For this review, take the finished solid that the model builds, in its own axes (mm). A direction names the side the tool comes from. Round coordinates to 2 decimals unless told otherwise and drop trailing zeros. Order: outer loops, then holes, each group sorted by start corner. A loop starts at its lowest first (then second) coordinate and runs counter-clockwise, first axis right, second up. Notation, with made-up numbers: (-26.5, 49) -> (8.5, 49) arc R14 cw to (8.5, 71) -> close; hole circle Ø8 at (67.5, 22). An arc over 180 degrees is marked (long way). Use a Markdown table: item, result. Add a question column.
1) Consider section A-A (y = -2.5). State the section outline as (x, z) points, plus the area to 3 significant figures.
2) Draft analysis for pull direction Z (two halves, no side actions). For faces 6 (the face through (11.37, -7.28, -23.12)), 7 (the face through (2, -23, -26)), 8 (the face through (8.819, -9.311, -24.174)), state which applies: pulls with the +Z half, pulls with the -Z half, needs draft (parallel to the pull), parting line crosses it, or undercut.
3) Clearance check with flat-ended pins moving along their axes: P1, Ø11, axis at x = -7, z = -2.5, coming from the -Y side; P2, Ø3, axis at y = -0.5, z = -16.5, coming from the -X side; P3, Ø1.9, axis at x = 6.5, z = -25.5, coming from the -Y side; P4, Ø8, axis at x = -16, z = -20.5, coming from the -Y side. State where each tip first meets the part, or that it passes through.
4) Machinability: for faces 1 (the face through (10, -23, -24)), 2 (the face through (13, 0, -13)), 3 (the face through (17, 8, 4)), 4 (the face through (9.63, -11.34, -22.53)), 5 (the face through (-7, -10, 16)), which of the approach directions +Z, -Z, +X, -X, +Y, -Y give a long, thin tool a straight path to every point of the face, cutting with its end or side? Answer none if there is none.
5) Consider section B-B (z = 0). State the section outline as (x, y) points.
6) Wall thickness on line 1 along X through (y, z) = (3.75, 0); line 2 along X through (y, z) = (-4, 0); line 3 along Y through (x, z) = (19, -13.5): over which ranges is each line inside the solid? List them lowest first. Write a range as [from, to].
7) Consider section C-C (x = -16). State the section outline as (y, z) points, plus the area to 3 significant figures.
```python
from build123d import *

# Parameters (mm, degrees)
SKETCH1_R           = 24.5
SKETCH1_R_2         = 18
SKETCH1_R_3         = 17.1
BOSS_EXTRUDE1_DEPTH = 8
SKETCH1_3_R         = 18
SKETCH1_3_R_2       = 17.1
BOSS_EXTRUDE2_DEPTH = 10
BOSS_EXTRUDE3_DEPTH = 4
BOSS_EXTRUDE4_DEPTH = 27


with BuildPart() as part:
    # Sketch1 → Boss-Extrude1 (new body)
    with BuildSketch(Plane(origin=(0, 0, 0), x_dir=(1, 0, 0), z_dir=(0, 1, 0))):
        with Locations(Location((0, 0, 0), (0, 0, 270))):
            Circle(SKETCH1_R)
        Circle(SKETCH1_R_2, mode=Mode.SUBTRACT)
        Circle(SKETCH1_R_2)
        with Locations(Location((0, 0, 0), (0, 0, 270))):
            Circle(SKETCH1_R_3, mode=Mode.SUBTRACT)
    extrude(amount=BOSS_EXTRUDE1_DEPTH)

    # Sketch1_3 → Boss-Extrude2 (add)
    with BuildSketch(Plane(origin=(0, 0, 0), x_dir=(1, 0, 0), z_dir=(0, 1, 0))):
        with Locations(Location((0, 0, 0), (0, 0, 270))):
            Circle(SKETCH1_3_R)
        with Locations(Location((0, 0, 0), (0, 0, 270))):
            Circle(SKETCH1_3_R_2, mode=Mode.SUBTRACT)
    extrude(amount=-BOSS_EXTRUDE2_DEPTH)

    # Sketch2 → Boss-Extrude3 (add)
    with BuildSketch(Plane(origin=(0, 8, 0), x_dir=(1, 0, 0), z_dir=(0, 1, 0))):
        with BuildLine():
            Line((0.558039299, 26.994232572), (0.506368994, 24.494766593))
            ThreePointArc((0.506368994, 24.494766593), (5.796003851, 23.804544511), (10.810861841, 21.985796921))
            Line((10.810861841, 21.985796921), (11.914011009, 24.229245586))
            ThreePointArc((11.914011009, 24.229245586), (6.387432816, 26.233579665), (0.558039299, 26.994232572))
        make_face()
    extrude(amount=-BOSS_EXTRUDE3_DEPTH)

    # Sketch3 → Boss-Extrude4 (add)
    with BuildSketch(Plane.XZ.offset(-4)):
        with BuildLine():
            Line((0.506368994, -24.494766593), (0.558039299, -26.994232572))
            ThreePointArc((0.558039299, -26.994232572), (2.171691116, -26.912520463), (3.777566106, -26.734434617))
            Line((3.777566106, -26.734434617), (3.427791467, -24.259024005))
            ThreePointArc((3.427791467, -24.259024005), (1.970608605, -24.420620421), (0.506368994, -24.494766593))
        make_face()
        with BuildLine():
            Line((8.396620698, -23.016228207), (9.253418728, -25.364822922))
            ThreePointArc((9.253418728, -25.364822922), (10.598934115, -24.832692073), (11.914011009, -24.229245586))
            Line((11.914011009, -24.229245586), (10.810861841, -21.985796921))
            ThreePointArc((10.810861841, -21.985796921), (9.617551327, -22.533368733), (8.396620698, -23.016228207))
        make_face()
    extrude(amount=BOSS_EXTRUDE4_DEPTH)


solid = part.part
```
Results list:
| question | item | result |
|---|---|---|
| 1 | outline | circle Ø36 at (0, 0); (0.51, -24.49) -> (0.56, -26.99) arc R27 ccw to (3.78, -26.73) -> (3.43, -24.26) arc R24.5 cw to start; (8.4, -23.02) -> (9.25, -25.36) arc R27 ccw to (11.91, -24.23) -> (10.81, -21.99) arc R24.5 cw to start; hole circle Ø34.2 at (0, 0) |
| 1 | area | 114 mm2 |
| 2 | face 6 | undercut |
| 2 | face 7 | needs draft |
| 2 | face 8 | pulls with the -Z half |
| 3 | P1 | through |
| 3 | P2 | x = -19.3 |
| 3 | P3 | y = 4 |
| 3 | P4 | y = 0 |
| 4 | face 1 | +Z, -Z, +X, -X, -Y |
| 4 | face 2 | -Y |
| 4 | face 3 | +Z, -Z, +X, -X, +Y |
| 4 | face 4 | -X, -Y |
| 4 | face 5 | +Z, +X, -X, -Y |
| 5 | outline | (-24.5, 0) -> (-18, 0) -> (-18, -10) -> (-17.1, -10) -> (-17.1, 8) -> (-24.5, 8) -> close; (17.1, -10) -> (18, -10) -> (18, 0) -> (24.5, 0) -> (24.5, 8) -> (17.1, 8) -> close |
| 6 | line 1 | [-24.5, -17.1], [17.1, 24.5] |
| 6 | line 2 | [-18, -17.1], [17.1, 18] |
| 6 | line 3 | [0, 8] |
| 7 | outline | (-10, -8.25) -> (0, -8.25) -> (0, -18.55) -> (8, -18.55) -> (8, -6.03) -> (-10, -6.03) -> close; (-10, 6.03) -> (8, 6.03) -> (8, 18.55) -> (0, 18.55) -> (0, 8.25) -> (-10, 8.25) -> close |
| 7 | area | 245 mm2 |
